```python
from build123d import *

# Parameters (mm, degrees)
SCHIZZO1_W                       = 6.5
SCHIZZO1_H                       = 6
BASE_FLANGIA1_DEPTH              = 0.5
BORDO_FLANGIA1_STRIP_W           = 2.4
BORDO_FLANGIA1_STRIP_H           = 0.5
BORDO_FLANGIA1_STRIP_CUT_DEPTH   = 6
BORDO_FLANGIA1_STRIP_2_W         = 2.4
BORDO_FLANGIA1_STRIP_2_H         = 0.5
BORDO_FLANGIA1_STRIP_CUT_2_DEPTH = 6
BORDO_FLANGIA1_DEPTH             = 6
BORDO_FLANGIA1_BEND_DEPTH        = 6
BORDO_FLANGIA2_STRIP_W           = 2.4
BORDO_FLANGIA2_STRIP_H           = 0.5
BORDO_FLANGIA2_STRIP_CUT_DEPTH   = 6
BORDO_FLANGIA2_STRIP_2_W         = 2.4
BORDO_FLANGIA2_STRIP_2_H         = 0.5
BORDO_FLANGIA2_STRIP_CUT_2_DEPTH = 6
BORDO_FLANGIA2_DEPTH             = 6
BORDO_FLANGIA2_BEND_DEPTH        = 6
SCHIZZO18_R                      = 0.75
TAGLIO_ESTRUSIONE1_DEPTH         = 14.921655792
SCHIZZO22_R                      = 0.75
TAGLIO_ESTRUSIONE2_DEPTH         = 14.921655792


# Sheet-metal steps are written as plain solids
with BuildPart() as part:
    # Schizzo1 → Base-Flangia1 (new body)
    with BuildSketch(Plane.XY):
        Rectangle(SCHIZZO1_W, SCHIZZO1_H)
    extrude(amount=-BASE_FLANGIA1_DEPTH)

    # Bordo-Flangia1 strip (across the edge) → Bordo-Flangia1 strip cut (cut)
    with BuildSketch(Plane(origin=(-3.25, -3, -0.5), x_dir=(1, 0, 0), z_dir=(0, 1, 0))):
        with Locations((-1, -0.25)):
            Rectangle(BORDO_FLANGIA1_STRIP_W, BORDO_FLANGIA1_STRIP_H)
    extrude(amount=BORDO_FLANGIA1_STRIP_CUT_DEPTH, mode=Mode.SUBTRACT)

    # Bordo-Flangia1 strip 2 (across the edge) → Bordo-Flangia1 strip cut 2 (cut)
    with BuildSketch(Plane(origin=(3.25, 3, -0.5), x_dir=(-1, 0, 0), z_dir=(0, -1, 0))):
        with Locations((-1, -0.25)):
            Rectangle(BORDO_FLANGIA1_STRIP_2_W, BORDO_FLANGIA1_STRIP_2_H)
    extrude(amount=BORDO_FLANGIA1_STRIP_CUT_2_DEPTH, mode=Mode.SUBTRACT)

    # Bordo-Flangia1 section (across the edge) → Bordo-Flangia1 (add)
    with BuildSketch(Plane(origin=(-3.25, -3, -0.5), x_dir=(1, 0, 0), z_dir=(0, 1, 0))):
        with BuildLine():
            Line((-0.5, 0.2), (-0.5, 11))
            Line((-0.5, 11), (0, 11))
            Line((0, 11), (0, 0.2))
            ThreePointArc((0, 0.2), (0.058578644, 0.058578644), (0.2, 0))
            Line((0.2, 0), (0.2, -0.5))
            ThreePointArc((0.2, -0.5), (-0.294974747, -0.294974747), (-0.5, 0.2))
        make_face()
    extrude(amount=BORDO_FLANGIA1_DEPTH)

    # Bordo-Flangia1 section 2 (across the edge) → Bordo-Flangia1 bend (add)
    with BuildSketch(Plane(origin=(3.25, 3, -0.5), x_dir=(-1, 0, 0), z_dir=(0, -1, 0))):
        with BuildLine():
            Line((-0.5, 0.2), (-0.5, 11))
            Line((-0.5, 11), (0, 11))
            Line((0, 11), (0, 0.2))
            ThreePointArc((0, 0.2), (0.058578644, 0.058578644), (0.2, 0))
            Line((0.2, 0), (0.2, -0.5))
            ThreePointArc((0.2, -0.5), (-0.294974747, -0.294974747), (-0.5, 0.2))
        make_face()
    extrude(amount=BORDO_FLANGIA1_BEND_DEPTH)

    # Bordo-Flangia2 strip (across the edge) → Bordo-Flangia2 strip cut (cut)
    with BuildSketch(Plane(origin=(-3.75, 3, -11.5), x_dir=(0, 0, 1), z_dir=(0, -1, 0))):
        with Locations((-1, -0.25)):
            Rectangle(BORDO_FLANGIA2_STRIP_W, BORDO_FLANGIA2_STRIP_H)
    extrude(amount=BORDO_FLANGIA2_STRIP_CUT_DEPTH, mode=Mode.SUBTRACT)

    # Bordo-Flangia2 strip 2 (across the edge) → Bordo-Flangia2 strip cut 2 (cut)
    with BuildSketch(Plane(origin=(3.75, -3, -11.5), x_dir=(0, 0, 1), z_dir=(0, 1, 0))):
        with Locations((-1, -0.25)):
            Rectangle(BORDO_FLANGIA2_STRIP_2_W, BORDO_FLANGIA2_STRIP_2_H)
    extrude(amount=BORDO_FLANGIA2_STRIP_CUT_2_DEPTH, mode=Mode.SUBTRACT)

    # Bordo-Flangia2 section (across the edge) → Bordo-Flangia2 (add)
    with BuildSketch(Plane(origin=(-3.75, 3, -11.5), x_dir=(0, 0, 1), z_dir=(0, -1, 0))):
        with BuildLine():
            Line((-0.5, 0.2), (-0.5, 3.5))
            Line((-0.5, 3.5), (0, 3.5))
            Line((0, 3.5), (0, 0.2))
            ThreePointArc((0, 0.2), (0.058578644, 0.058578644), (0.2, 0))
            Line((0.2, 0), (0.2, -0.5))
            ThreePointArc((0.2, -0.5), (-0.294974747, -0.294974747), (-0.5, 0.2))
        make_face()
    extrude(amount=BORDO_FLANGIA2_DEPTH)

    # Bordo-Flangia2 section 2 (across the edge) → Bordo-Flangia2 bend (add)
    with BuildSketch(Plane(origin=(3.75, -3, -11.5), x_dir=(0, 0, 1), z_dir=(0, 1, 0))):
        with BuildLine():
            Line((-0.5, 0.2), (-0.5, 3.5))
            Line((-0.5, 3.5), (0, 3.5))
            Line((0, 3.5), (0, 0.2))
            ThreePointArc((0, 0.2), (0.058578644, 0.058578644), (0.2, 0))
            Line((0.2, 0), (0.2, -0.5))
            ThreePointArc((0.2, -0.5), (-0.294974747, -0.294974747), (-0.5, 0.2))
        make_face()
    extrude(amount=BORDO_FLANGIA2_BEND_DEPTH)

    # Schizzo18 → Taglio-Estrusione1 (cut, through all)
    with BuildSketch(Plane.XY.offset(-11.5)):
        with Locations((5.25, 0.75)):
            Circle(SCHIZZO18_R)
        with Locations((5.25, -1.75)):
            Circle(SCHIZZO18_R)
    extrude(amount=-TAGLIO_ESTRUSIONE1_DEPTH, mode=Mode.SUBTRACT)

    # Schizzo22 → Taglio-Estrusione2 (cut, through all)
    with BuildSketch(Plane.XY.offset(-11.5)):
        with Locations((-5.25, 1.75)):
            Circle(SCHIZZO22_R)
        with Locations((-5.25, -0.75)):
            Circle(SCHIZZO22_R)
    extrude(amount=-TAGLIO_ESTRUSIONE2_DEPTH, mode=Mode.SUBTRACT)


solid = part.part
```
The model under review builds one solid part; all positions refer to its coordinate system, in mm. A direction names the side the tool comes from. Round coordinates to 2 decimals unless told otherwise and drop trailing zeros. Loops run counter-clockwise (first coordinate to the right, second up) from the corner with the lowest first, then second, coordinate; pieces in that order, holes last.
Item 1: Take a section at D-D (y = -0.3). Write out the cut boundary in (x, z), then the cut area to 3 significant figures.
Determined:
outline: (-7.25, -12) - (-5.85, -12) - (-5.85, -11.5) - (-7.25, -11.5) - close; (-4.65, -12) - (-3.95, -12) arc R0.7 ccw to (-3.25, -11.3) - (-3.25, -0.7) arc R0.2 cw to (-3.05, -0.5) - (3.05, -0.5) arc R0.2 cw to (3.25, -0.7) - (3.25, -11.3) arc R0.7 ccw to (3.95, -12) - (7.25, -12) - (7.25, -11.5) - (3.95, -11.5) arc R0.2 cw to (3.75, -11.3) - (3.75, -0.7) arc R0.7 ccw to (3.05, 0) - (-3.05, 0) arc R0.7 ccw to (-3.75, -0.7) - (-3.75, -11.3) arc R0.2 cw to (-3.95, -11.5) - (-4.65, -11.5) - close
area: 17.8 mm2
Item 2: Take a section at C-C (x = -5.25). Write out the cut boundary in (y, z).
Determined:
outline: (-3, -12) - (-1.5, -12) - (-1.5, -11.5) - (-3, -11.5) - close; (0, -12) - (1, -12) - (1, -11.5) - (0, -11.5) - close; (2.5, -12) - (3, -12) - (3, -11.5) - (2.5, -11.5) - close
Item 3: Clearance check with flat-ended pins moving along their axes: pin 1 Ø5 at (x, z) = (0, -8.5) entering from -Y; pin 2 Ø3 at (y, z) = (1, -8.5) entering from -X; pin 3 Ø2.5 at (x, y) = (5.5, 0) entering from +Z; pin 4 Ø2 at (y, z) = (0, -3) entering from +X. State where each tip first meets the part, or that it passes through.
Determined:
pin 1: passes through
pin 2: stops at x = -3.75
pin 3: stops at z = -11.5
pin 4: stops at x = 3.75
Item 4: For line 1 (Y direction, x = -5.25, z = -11.9); line 2 (X direction, y = -0.6, z = -3.5); line 3 (Y direction, x = 5.25, z = -11.8), list the stretches that pass through material, from the lowest coordinate up.
Determined:
line 1: y = -3 to -1.5, 0 to 1, 2.5 to 3
line 2: x = -3.75 to -3.25, 3.25 to 3.75
line 3: y = -3 to -2.5, -1 to 0, 1.5 to 3
Item 5: For faces 1 (the face through (3.75, 0, -6)), 2 (the face through (3.25, 0, -6)), 3 (the face through (-6, 0, -11.5)), 4 (the face through (4.7, -1.24, -11.75)), list the 3-axis set-ups (+Z, -Z, +X, -X, +Y, -Y) from which the entire face can be reached by the end or side of a thin tool; tool diameter is ignored.
Determined:
face 1: +Z, +X, +Y, -Y
face 2: -Z, +Y, -Y
face 3: +Z, -X, +Y, -Y
face 4: +Z, -Z
Item 6: Mouldability with a two-part tool opening along X and no side actions: class faces 5 (the face through (-3.25, 0, -6)), 6 (the face through (-3.75, 0, -6)), 7 (the face through (6, 0, -11.5)) as released by +X, released by -X, zero draft, split by the parting line, or undercut.
Determined:
face 5: undercut
face 6: released by -X
face 7: zero draft
Item 7: Take a section at B-B (z = -9). Write out the cut boundary in (x, y), then the cut area to 3 significant figures.
Determined:
outline: (-3.75, -3) - (-3.25, -3) - (-3.25, 3) - (-3.75, 3) - close; (3.25, -3) - (3.75, -3) - (3.75, 3) - (3.25, 3) - close
area: 6.00 mm2
Item 8: Take a section at A-A (y = 0.75). Write out the cut boundary in (x, z), then the cut area to 3 significant figures.
Determined:
outline: (-7.25, -12) - (-3.95, -12) arc R0.7 ccw to (-3.25, -11.3) - (-3.25, -0.7) arc R0.2 cw to (-3.05, -0.5) - (3.05, -0.5) arc R0.2 cw to (3.25, -0.7) - (3.25, -11.3) arc R0.7 ccw to (3.95, -12) - (4.5, -12) - (4.5, -11.5) - (3.95, -11.5) arc R0.2 cw to (3.75, -11.3) - (3.75, -0.7) arc R0.7 ccw to (3.05, 0) - (-3.05, 0) arc R0.7 ccw to (-3.75, -0.7) - (-3.75, -11.3) arc R0.2 cw to (-3.95, -11.5) - (-7.25, -11.5) - close; (6, -12) - (7.25, -12) - (7.25, -11.5) - (6, -11.5) - close
area: 17.6 mm2
